```python
from build123d import *

# Parameters (mm, degrees)
ESBO_O1_W                  = 180
ESBO_O1_H                  = 65
RESSALTO_EXTRUS_O2_DEPTH   = 32.5
FILETE1_R                  = 33
CORTE_EXTRUS_O1_DEPTH      = 102.056914657
CORTE_EXTRUS_O1_DEPTH_BACK = 102.056914657
ESBO_O2_W                  = 65
ESBO_O2_H                  = 35
FILETE4_R                  = 33
ESBO_O4_W                  = 65
ESBO_O4_H                  = 35
CORTE_EXTRUS_O2_DEPTH      = 116.674405799
ESBO_O5_R                  = 10
CORTE_EXTRUS_O3_DEPTH      = 116.674405799
ESBO_O6_R                  = 10
CORTE_EXTRUS_O4_DEPTH      = 116.674405799


with BuildPart() as part:
    # Esboço1 → Ressalto-extrusão2 (new, symmetric)
    with BuildSketch(Plane.XY):
        Rectangle(ESBO_O1_W, ESBO_O1_H)
    extrude(amount=RESSALTO_EXTRUS_O2_DEPTH, both=True)

    # Filete1
    # the kernel refuses this fillet: 33 mm, written as the material it takes off along each edge
    with BuildSketch(Plane(origin=(-90, -115, 32.5), x_dir=(1, 0, 0), z_dir=(0, 1, 0))) as filete1_piece_1:
        with BuildLine():
            CenterArc((FILETE1_R, FILETE1_R), FILETE1_R, 180, 90)
            Line((0, FILETE1_R), (0, 0))
            Line((0, 0), (FILETE1_R, 0))
        make_face()
    extrude(amount=230, mode=Mode.SUBTRACT)
    with BuildSketch(Plane(origin=(-90, -115, -32.5), x_dir=(1, 0, 0), z_dir=(0, 1, 0))) as filete1_piece_2:
        with BuildLine():
            CenterArc((FILETE1_R, -FILETE1_R), FILETE1_R, 90, 90)
            Line((0, -FILETE1_R), (0, 0))
            Line((0, 0), (FILETE1_R, 0))
        make_face()
    extrude(amount=230, mode=Mode.SUBTRACT)

    # Esboço2 → Corte-extrusão1 (cut, two sides: drawn at the far end of the back side and taken through both)
    with BuildSketch(Plane.XY.offset(-CORTE_EXTRUS_O1_DEPTH_BACK)):
        with Locations((-57.496211904, 0)):
            Rectangle(ESBO_O2_W, ESBO_O2_H)
    extrude(amount=CORTE_EXTRUS_O1_DEPTH + CORTE_EXTRUS_O1_DEPTH_BACK, mode=Mode.SUBTRACT)

    # Filete4
    # the kernel refuses this fillet: 33 mm, written as the material it takes off along each edge
    with BuildSketch(Plane(origin=(90, -32.5, 115), x_dir=(0, 1, 0), z_dir=(0, 0, -1)), Plane(origin=(90, 32.5, 115), x_dir=(-1, 0, 0), z_dir=(0, 0, -1))) as filete4_piece_1:
        with BuildLine():
            CenterArc((FILETE4_R, -FILETE4_R), FILETE4_R, 90, 90)
            Line((0, -FILETE4_R), (0, 0))
            Line((0, 0), (FILETE4_R, 0))
        make_face()
    extrude(amount=230, mode=Mode.SUBTRACT)

    # Esboço4 → Corte-extrusão2 (cut, through all)
    with BuildSketch(Plane(origin=(0, 32.5, 0), x_dir=(1, 0, 0), z_dir=(0, 1, 0))):
        with Locations((57.496211904, 0)):
            Rectangle(ESBO_O4_W, ESBO_O4_H)
    extrude(amount=-CORTE_EXTRUS_O2_DEPTH, mode=Mode.SUBTRACT)

    # Esboço5 → Corte-extrusão3 (cut, through all)
    with BuildSketch(Plane(origin=(0, 0, -32.5), x_dir=(-1, 0, 0), z_dir=(0, 0, -1))):
        with Locations((-57, -0.5)):
            Circle(ESBO_O5_R)
    extrude(amount=-CORTE_EXTRUS_O3_DEPTH, mode=Mode.SUBTRACT)

    # Esboço6 → Corte-extrusão4 (cut, through all)
    with BuildSketch(Plane(origin=(0, 32.5, 0), x_dir=(1, 0, 0), z_dir=(0, 1, 0))):
        with Locations(Location((-57, -0.5, 0), (0, 0, 270))):
            Circle(ESBO_O6_R)
    extrude(amount=-CORTE_EXTRUS_O4_DEPTH, mode=Mode.SUBTRACT)


solid = part.part
```
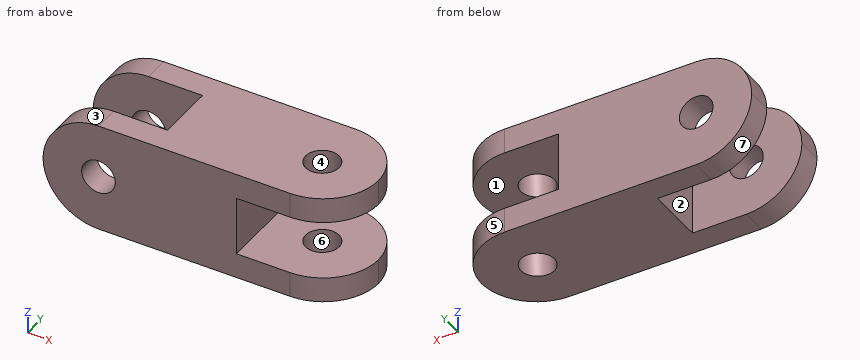
Input: part model. Units: mm. Frame: model coordinates. Face numbers are marked on the shaded views. A direction names the side the tool comes from. Give positions to 0.01 mm unless a question says otherwise; leave off trailing zeros. Order: outer loops, then holes, each group sorted by start corner. A loop starts at its lowest first (then second) coordinate and runs counter-clockwise, first axis right, second up. Notation, with made-up numbers: M -40,31.5 L -13,31.5 A14 cw -13,58.5 Z; hole C 7,59.5 d9. An arc over 180 degrees is marked long. Return JSON: item names as keys, results as strings.
Item 1: Cut plane C-C (y = -24). Return loops of the section in (x, z), then the cut area to 3 significant figures.
Solutions:
{"outline": "M -90,0 A33 ccw -57,-32.5 L 79.11,-32.5 L 79.11,-17.5 L 25,-17.5 L 25,17.5 L 79.11,17.5 L 79.11,32.5 L -57,32.5 A33 ccw Z; hole C -57,0.5 d20", "area": "8,320 mm^2"}
Item 2: First-contact query: P1, Ø16, axis at x = -57, z = 0.5, coming from the +Y side; P2, Ø23, axis at x = -57, z = 0.5, coming from the +Y side; P3, Ø2, axis at y = -13, z = -6, coming from the +X side. Flat tips, straight axial feed; report the tip coordinate or a pass-through.
Solutions:
{"P1": "through", "P2": "y = 32.5", "P3": "x = 25"}
Item 3: Ray query, probe 1 along X at (y, z) = (29.25, 0.5); probe 2 along Y at (x, z) = (57, -26); probe 3 along Y at (x, z) = (-71, -1). Return the intervals inside material, ascending.
Solutions:
{"probe 1": "-89.98 to -67, -47 to 25", "probe 2": "-32.5 to -10.5, 9.5 to 32.5", "probe 3": "-32.5 to -17.5, 17.5 to 32.5"}
Item 4: Cut plane D-D (z = 4). Return loops of the section in (x, y).
Solutions:
{"outline": "M -89.69,-32.5 L -66.37,-32.5 L -66.37,-17.5 L -89.69,-17.5 Z; M -89.69,17.5 L -66.37,17.5 L -66.37,32.5 L -89.69,32.5 Z; M -47.63,-32.5 L 25,-32.5 L 25,32.5 L -47.63,32.5 L -47.63,17.5 L -25,17.5 L -25,-17.5 L -47.63,-17.5 Z"}
Item 5: Cut plane B-B (z = -23). Return loops of the section in (x, y), then the cut area to 3 significant figures.
Solutions:
{"outline": "M -80.17,-32.5 L 57,-32.5 A33 ccw 90,0 A33 ccw 57,32.5 L -80.17,32.5 L -80.17,17.5 L -25,17.5 L -25,-17.5 L -80.17,-17.5 Z; hole C 57,-0.5 d20", "area": "8,350 mm^2"}
Item 6: Cut plane A-A (x = -52). Return loops of the section in (y, z), then the cut area to 3 significant figures.
Solutions:
{"outline": "M -32.5,-32.5 L -17.5,-32.5 L -17.5,-8.16 L -32.5,-8.16 Z; M -32.5,9.16 L -17.5,9.16 L -17.5,32.5 L -32.5,32.5 Z; M 17.5,-32.5 L 32.5,-32.5 L 32.5,-8.16 L 17.5,-8.16 Z; M 17.5,9.16 L 32.5,9.16 L 32.5,32.5 L 17.5,32.5 Z", "area": "1,430 mm^2"}
Item 7: Access query for the marked faces 1, 2 and 3. Directions: +Z, -Z, +X, -X, +Y, -Y. A direction counts if a zero-diameter tool reaches every point of the face in a straight line with its end or side. Return the directions, or none.
Solutions:
{"face 1": "+X, +Y, -Y", "face 2": "+Z, -Z, -X", "face 3": "+Z, -X, +Y, -Y"}
Item 8: Pull-direction query (Y, two-part tool) for the marked faces 4, 5, 6 and 7; classes: +Y half, -Y half, draft (parallel to the pull), parting line (faces both ways), or undercut.
Solutions:
{"face 4": "undercut", "face 5": "+Y half", "face 6": "undercut", "face 7": "draft"}
